from build123d import *

# Parameters (mm, degrees)
SKETCH1_R           = 28.5
SKETCH1_R_2         = 21
BOSS_EXTRUDE1_DEPTH = 13.175
SKETCH2_R           = 2.25
CUT_EXTRUDE1_DEPTH  = 43.403780787
CIRPATTERN1_COUNT   = 4
SKETCH3_R           = 2.25
CUT_EXTRUDE2_DEPTH  = 49.154153681


with BuildPart() as part:
    # Sketch1 → Boss-Extrude1 (new, symmetric)
    with BuildSketch(Plane(origin=(0, 0, 0), x_dir=(1, 0, 0), z_dir=(0, 1, 0))):
        with Locations(Location((0, 0, 0), (0, 0, 90))):
            Circle(SKETCH1_R)
        with Locations(Location((0, 0, 0), (0, 0, 90))):
            Circle(SKETCH1_R_2, mode=Mode.SUBTRACT)
    extrude(amount=BOSS_EXTRUDE1_DEPTH, both=True)

    # Sketch2 → Cut-Extrude1 (cut, through all)
    with BuildSketch(Plane.XY):
        with Locations(Location((0, 8.175, 0), (0, 0, 90))):
            Circle(SKETCH2_R)
        with Locations(Location((0, -8.175, 0), (0, 0, 90))):
            Circle(SKETCH2_R)
    cut_extrude1 = extrude(amount=-CUT_EXTRUDE1_DEPTH, mode=Mode.SUBTRACT)

    # CirPattern1: Cut-Extrude1 ×4 about axis
    cirpattern1_axis = Axis((0, 13.175, 0), (0, -1, 0))
    for i in range(1, CIRPATTERN1_COUNT):
        add(cut_extrude1.rotate(cirpattern1_axis, i * 360 / CIRPATTERN1_COUNT), mode=Mode.SUBTRACT)

    # Sketch3 → Cut-Extrude2 (cut, through all)
    with BuildSketch(Plane(origin=(0, 13.175, 0), x_dir=(1, 0, 0), z_dir=(0, 1, 0))):
        with Locations(Location((17.500892834, 17.500892834, 0), (0, 0, 270))):
            Circle(SKETCH3_R)
        with Locations(Location((17.500892834, -17.500892834, 0), (0, 0, 270))):
            Circle(SKETCH3_R)
        with Locations(Location((-17.500892834, -17.500892834, 0), (0, 0, 270))):
            Circle(SKETCH3_R)
        with Locations(Location((-17.500892834, 17.500892834, 0), (0, 0, 270))):
            Circle(SKETCH3_R)
    extrude(amount=-CUT_EXTRUDE2_DEPTH, mode=Mode.SUBTRACT)


solid = part.part
Input: part model. Units: mm. Frame: model coordinates. Give positions to 0.01 mm unless a question says otherwise; leave off trailing zeros. Order: outer loops, then holes, each group sorted by start corner. A loop starts at its lowest first (then second) coordinate and runs counter-clockwise, first axis right, second up. Notation, with made-up numbers: (25.5, -23.5) - (33.5, -23.5) arc R17 cw to (33.5, -5.5) - close; hole circle Ø1 at (-8, 87.5). An arc over 180 degrees is marked (long way). Answer as a JSON object with one key per item and string values. Group by question number.
Q1. Cut plane A-A, the plane y = 9.25. Output: boundary loops of the cut face in (x, z), then the cut area to 3 significant figures.
Q2. Cut plane D-D, the plane z = 8. Output: boundary loops of the cut face in (x, y) (3 decimals).
Q3. First-contact query: pin 1 Ø2 at (x, y) = (-14.5, 8) entering from -Z; pin 2 Ø12 at (x, y) = (-11, 7.5) entering from +Z; pin 3 Ø8 at (x, z) = (10.5, -17.5) entering from +Y (3 decimals); pin 4 Ø4 at (x, y) = (-21.5, 1) entering from -Z. Flat tips, straight axial feed; report the tip coordinate or a pass-through.
Q4. Cut plane B-B, the plane z = 0. Output: boundary loops of the cut face in (x, y) (3 decimals), then the cut area to 3 significant figures.
Q5. Line query: probe 1 along X at (y, z) = (-9.5, 17.5); probe 2 along Z at (x, y) = (-17, 3.25); probe 3 along Z at (x, y) = (-18, -7.5). Output: solid intervals per line, ascending.
Q6. Mould query, pull axis X, two halves, no side actions, for faces 1 (the face through (10.916, 0.184, -26.327)), 2 (the face through (-6.31, -0.18, -20.03)), 3 (the face through (21, -13.175, 4)). Classes: pulls with the +X half, pulls with the -X half, needs draft (parallel to the pull), parting line crosses it, or undercut.
Q7. Cut plane C-C, the plane x = 0. Output: boundary loops of the cut face in (y, z) (3 decimals), then the cut area to 3 significant figures.
Results:
{
 "1": {"outline": "(-28.43, -1.98) arc R28.5 ccw to (-1.98, -28.43) - (-1.98, -20.91) arc R21 cw to (-20.91, -1.98) - close; (-28.43, 1.98) - (-20.91, 1.98) arc R21 cw to (-1.98, 20.91) - (-1.98, 28.43) arc R28.5 ccw to start; (1.98, -28.43) arc R28.5 ccw to (28.43, -1.98) - (20.91, -1.98) arc R21 cw to (1.98, -20.91) - close; (1.98, 20.91) arc R21 cw to (20.91, 1.98) - (28.43, 1.98) arc R28.5 ccw to (1.98, 28.43) - close; hole circle Ø4.5 at (-17.5, -17.5); hole circle Ø4.5 at (-17.5, 17.5); hole circle Ø4.5 at (17.5, -17.5); hole circle Ø4.5 at (17.5, 17.5)", "area": "984 mm^2"},
 "2": {"outline": "(-27.354, -13.175) - (-19.416, -13.175) - (-19.416, 13.175) - (-27.354, 13.175) - close; (19.416, -13.175) - (27.354, -13.175) - (27.354, 13.175) - (19.416, 13.175) - close"},
 "3": {"pin 1": "z = -25.1", "pin 2": "z = 28.06", "pin 3": "y = 13.175", "pin 4": "z = -20.78"},
 "4": {"outline": "(-28.5, -13.175) - (-21, -13.175) - (-21, -10.425) - (-28.5, -10.425) - close; (-28.5, -5.925) - (-21, -5.925) - (-21, 5.925) - (-28.5, 5.925) - close; (-28.5, 10.425) - (-21, 10.425) - (-21, 13.175) - (-28.5, 13.175) - close; (21, -13.175) - (28.5, -13.175) - (28.5, -10.425) - (21, -10.425) - close; (21, -5.925) - (28.5, -5.925) - (28.5, 5.925) - (21, 5.925) - close; (21, 10.425) - (28.5, 10.425) - (28.5, 13.175) - (21, 13.175) - close", "area": "260 mm^2"},
 "5": {"probe 1": "-22.49 to -19.75, -15.25 to -11.61, 11.61 to 15.25, 19.75 to 22.49", "probe 2": "-22.87 to -19.69, -15.31 to -12.33, 12.33 to 15.31, 19.69 to 22.87", "probe 3": "-22.1 to -19.69, -15.31 to -10.82, 10.82 to 15.31, 19.69 to 22.1"},
 "6": {"face 1": "parting line crosses it", "face 2": "undercut", "face 3": "needs draft"},
 "7": {"outline": "(-13.175, -28.5) - (-10.425, -28.5) - (-10.425, -21) - (-13.175, -21) - close; (-13.175, 21) - (-10.425, 21) - (-10.425, 28.5) - (-13.175, 28.5) - close; (-5.925, -28.5) - (5.925, -28.5) - (5.925, -21) - (-5.925, -21) - close; (-5.925, 21) - (5.925, 21) - (5.925, 28.5) - (-5.925, 28.5) - close; (10.425, -28.5) - (13.175, -28.5) - (13.175, -21) - (10.425, -21) - close; (10.425, 21) - (13.175, 21) - (13.175, 28.5) - (10.425, 28.5) - close", "area": "260 mm^2"}
}
